Can you work these out from the model? Positions are in its coordinate system, mm. Give positions to 0.01 mm unless a question says otherwise; leave off trailing zeros. Write each loop counter-clockwise with the first axis right and the second up, starting at its lowest first coordinate (ties: lowest second). Pieces come first, ordered by that corner, then holes. Notation, with made-up numbers: M -34.75,53.5 L 6.25,53.5 A37 ccw 6.25,90.5 Z; hole C 4.25,9 d9. An arc over 180 degrees is marked long. Write each question's results on one line, items separated by ' | '.
from build123d import *

# Parameters (mm, degrees)
SKETCH2_W           = 42.5
SKETCH2_H           = 15
SKETCH2_R           = 1
BOSS_EXTRUDE1_DEPTH = 2.3
FILLET9_R           = 10
SKETCH3_R           = 1
CUT_EXTRUDE1_DEPTH  = 3.3


with BuildPart() as part:
    # Sketch2 → Boss-Extrude1 (new body)
    with BuildSketch(Plane(origin=(0, 0, 0), x_dir=(1, 0, 0), z_dir=(0, 1, 0))):
        Rectangle(SKETCH2_W, SKETCH2_H)
        with Locations((0, -4.25)):
            Circle(SKETCH2_R, mode=Mode.SUBTRACT)
    extrude(amount=BOSS_EXTRUDE1_DEPTH)

    # Fillet9
    fillet9_edges = [part.edges().sort_by_distance(p)[0] for p in [
        (-21.25, 1.15, -7.5),
        (21.25, 1.15, -7.5),
    ]]
    fillet(fillet9_edges, radius=FILLET9_R)

    # Sketch3 → Cut-Extrude1 (cut, through all)
    with BuildSketch(Plane(origin=(0, 2.3, 0), x_dir=(1, 0, 0), z_dir=(0, 1, 0))):
        with Locations((0, -4.388678083)):
            Circle(SKETCH3_R)
    extrude(amount=-CUT_EXTRUDE1_DEPTH, mode=Mode.SUBTRACT)


solid = part.part
Item 1: I want a section at C-C, the plane y = 1.35. Please give me the cut outline in (x, z).
Geometry says:
outline: M -21.25,2.5 A10 ccw -11.25,-7.5 L 11.25,-7.5 A10 ccw 21.25,2.5 L 21.25,7.5 L -21.25,7.5 Z; hole M -1,4.32 A1 ccw long 1,4.32 A1 ccw long Z
Item 2: I want a section at A-A, the plane x = 0. Please give me the cut outline in (y, z), and give its area (3 significant figures).
Geometry says:
outline: M 0,-7.5 L 2.3,-7.5 L 2.3,3.25 L 0,3.25 Z; M 0,5.39 L 2.3,5.39 L 2.3,7.5 L 0,7.5 Z | area: 29.6 mm2
Item 3: Thinking about a two-plate mould opening in X: for faces 1 (the face through (21.25, 1, 5)), 2 (the face through (-0.02, 1.17, 5.39)), 3 (the face through (0, 1, -7.5)), which applies, +X half, -X half, draft (parallel to the pull), parting line (faces both ways), or undercut?
Geometry says:
face 1: +X half | face 2: undercut | face 3: draft
Item 4: If I drill on line 1 (X direction, y = 0.35, z = 2.25); line 2 (X direction, y = 2.15, z = 5.25); line 3 (X direction, y = 0.85, z = -2.5), over which ranges is the centre line in solid material (lowest first)? Write a range as from..to.
Geometry says:
line 1: x = -21.25..21.25 | line 2: x = -21.25..-0.51, 0.51..21.25 | line 3: x = -19.91..19.91
Item 5: I want a section at D-D, the plane z = -5.5. Please give me the cut outline in (x, y), and give its area (4 significant figures).
Geometry says:
outline: M -17.25,0 L 17.25,0 L 17.25,2.3 L -17.25,2.3 Z | area: 79.35 mm2
Item 6: I want a section at B-B, the plane z = 3.75. Please give me the cut outline in (x, y), and give its area (3 significant figures).
Geometry says:
outline: M -21.25,0 L -0.87,0 L -0.87,2.3 L -21.25,2.3 Z; M 0.87,0 L 21.25,0 L 21.25,2.3 L 0.87,2.3 Z | area: 93.8 mm2
Item 7: I'm going to push a flat-ended pin straight in: pin 1 (1 mm diameter, centred on y = 2, z = -3, fed in from +X). Where does the tip first touch, or does it pass through?
Geometry says:
pin 1: stops at x = 19.91
